Here's how the part is built. I have some questions about the finished solid (model axes, mm). A direction names the side the tool comes from. Coordinates: 2 decimals unless noted, no trailing zeros. Write each loop counter-clockwise with the first axis right and the second up, starting at its lowest first coordinate (ties: lowest second). Pieces come first, ordered by that corner, then holes. Notation, with made-up numbers: (-13, 74) - (27, 74) arc R11 cw to (27, 84) - close; hole circle Ø1 at (79, -7.5). An arc over 180 degrees is marked (long way). Answer in a Markdown table with one row per item. Add a question column.
Item 1: Imagine slicing it at C-C (x = 62.5). Please give me the cut outline in (y, z).
Item 2: Imagine slicing it at A-A (z = 0). Please give me the cut outline in (x, y), plus the area to 3 significant figures.
Item 3: I'm going to push flat-ended pins straight in: pin 1 (2 mm diameter, centred on y = -1.5, z = 1, fed in from +X); pin 2 (1 mm diameter, centred on x = 53.5, z = 2, fed in from +Y). Where does each tip first touch, or does it pass through?
Item 4: Which directions (+Z, -Z, +X, -X, +Y, -Y) give clear straight access to the entire face, cutting with the end or side of a thin tool? Please do faces 4 (the face through (-2.72, -1.5, -0.07)), 5 (the face through (75, 1, -1)), 6 (the face through (38.02, -0.9, 2.86)).
Item 5: If I drill on probe 1 along Z at (x, y) = (74, -1.5); probe 2 along X at (y, z) = (-1.8, 1.65); probe 3 along Z at (x, y) = (40.5, -0.2), over which ranges is the centre line in solid material (lowest first)? Write a range as from..to.
Item 6: We'd pull the mould along X, two halves only. Please class faces 1 (the face through (80, 0, 0)), 2 (the face through (75.49, 0.65, -1.01)), 3 (the face through (77.97, -1.5, -0.07)): +X half, -X half, draft (parallel to the pull), parting line (faces both ways), or undercut.
from build123d import *

# Parameters (mm, degrees)
SKETCH1_W     = 75
SKETCH1_H     = 3
CHAMFER1_SIZE = 0.4
SKETCH5_W     = 5
SKETCH5_H     = 1.5
FILLET3_R     = 0.5
CHAMFER4_SIZE = 0.4


with BuildPart() as part:
    # Sketch1 → Revolve1 (revolve)
    with BuildSketch(Plane.XY, mode=Mode.PRIVATE) as revolve1_sk:
        with Locations((37.5, 1.5)):
            Rectangle(SKETCH1_W, SKETCH1_H)
    revolve(revolve1_sk.sketch.rotate(Axis((0, 0, 0), (1, 0, 0)), 90), axis=Axis((0, 0, 0), (1, 0, 0)))

    # Chamfer1
    chamfer1_edges = [part.edges().sort_by_distance(p)[0] for p in [
        (0, 0, -3),
    ]]
    chamfer(chamfer1_edges, length=CHAMFER1_SIZE)

    # Sketch5 → Revolve4 (revolve)
    with BuildSketch(Plane.XY):
        Polygon((80, 0), (80, 1.5), (76, 1.5), (76, 1.2), (75, 1.2), (75, 0), align=None)
        with Locations((-2.5, 0.75)):
            Rectangle(SKETCH5_W, SKETCH5_H)
    revolve(axis=Axis((80, 0, 0), (-1, 0, 0)))

    # Fillet3
    fillet3_edges = [part.edges().sort_by_distance(p)[0] for p in [
        (0, -1.5, 0),
    ]]
    fillet(fillet3_edges, radius=FILLET3_R)

    # Chamfer4
    chamfer4_edges = [part.edges().sort_by_distance(p)[0] for p in [
        (75, 0, -3),
    ]]
    chamfer(chamfer4_edges, length=CHAMFER4_SIZE)


solid = part.part
Here are the results:
| question | item | result |
|---|---|---|
| 1 | outline | circle Ø6 at (0, 0) |
| 2 | outline | (-5, -1.5) - (-0.5, -1.5) arc R0.5 cw to (0, -2) - (0, -2.6) - (0.4, -3) - (74.6, -3) - (75, -2.6) - (75, -1.2) - (76, -1.2) - (76, -1.5) - (80, -1.5) - (80, 1.5) - (76, 1.5) - (76, 1.2) - (75, 1.2) - (75, 2.6) - (74.6, 3) - (0.4, 3) - (0, 2.6) - (0, 2) arc R0.5 cw to (-0.5, 1.5) - (-5, 1.5) - close |
| 2 | area | 479 mm2 |
| 3 | pin 1 | stops at x = 80 |
| 3 | pin 2 | stops at y = 2.6 |
| 4 | face 4 | -X |
| 4 | face 5 | none |
| 4 | face 6 | +X, -X |
| 5 | probe 1 | z = -2.6..2.6 |
| 5 | probe 2 | x = 0..75 |
| 5 | probe 3 | z = -2.99..2.99 |
| 6 | face 1 | +X half |
| 6 | face 2 | undercut |
| 6 | face 3 | draft |
